Geometry: final body of the model. Coordinates: model frame, mm. A direction names the side the tool comes from. Give positions to 0.01 mm unless a question says otherwise; leave off trailing zeros. Write each loop counter-clockwise with the first axis right and the second up, starting at its lowest first coordinate (ties: lowest second). Pieces come first, ordered by that corner, then holes. Notation, with made-up numbers: M -35,52.25 L -28,52.25 A25 cw -28,91.25 Z; hole C 25,65.25 d11. An arc over 180 degrees is marked long. Answer as a JSON object with one key per item and string values.
from build123d import *

# Parameters (mm, degrees)
F0_W     = 35.56
F0_H     = 35.56
F1_DEPTH = 5.08
F2_W     = 19.812
F2_H     = 4.572
F3_DEPTH = 2.54
F4_W     = 19.812
F4_H     = 4.572
F5_DEPTH = 2.54
F6_W     = 20.32
F6_H     = 5.08
F7_DEPTH = 2.54
F8_W     = 20.32
F8_H     = 5.08
F9_DEPTH = 2.54


with BuildPart() as f1:
    # F0 (on Top) → F1 (new body, symmetric)
    with BuildSketch(Plane.XY):
        Rectangle(F0_W, F0_H)
        Polygon((10.7597222222, 12.4850260417), (10.7597222222, -12.7), (5.4349826389, -12.7), (5.4349826389, -1.8300347222), (-4.5365017361, -1.8300347222), (-4.5365017361, -12.7), (-9.8777777778, -12.7), (-9.8777777778, 12.4850260417), (-4.5365017361, 12.4850260417), (-4.5365017361, 2.6127604167), (5.4349826389, 2.6127604167), (5.4349826389, 12.4850260417), align=None, mode=Mode.SUBTRACT)
    extrude(amount=F1_DEPTH, both=True)

    # F2 (on face) → F3 (join)
    with BuildSketch(Plane(origin=(0, 17.78, 0), x_dir=(-1, 0, 0), z_dir=(0, 1, 0))):
        Rectangle(F2_W, F2_H)
    extrude(amount=F3_DEPTH)

    # F4 (on face) → F5 (join)
    with BuildSketch(Plane(origin=(-17.78, 0, 0), x_dir=(0, -1, 0), z_dir=(-1, 0, 0))):
        Rectangle(F4_W, F4_H)
    extrude(amount=F5_DEPTH)

    # F6 (on face) → F7 (cut)
    with BuildSketch(Plane.XZ.offset(17.78)):
        Rectangle(F6_W, F6_H)
    extrude(amount=-F7_DEPTH, mode=Mode.SUBTRACT)

    # F8 (on face) → F9 (cut)
    with BuildSketch(Plane.YZ.offset(17.78)):
        Rectangle(F8_W, F8_H)
    extrude(amount=-F9_DEPTH, mode=Mode.SUBTRACT)


solid = f1.part
1) Cut plane D-D on y = 8.5. Return loops of the section in (x, z).
Geometry check:
{"outline": "M -20.32,-2.29 L -17.78,-2.29 L -17.78,-5.08 L -9.88,-5.08 L -9.88,5.08 L -17.78,5.08 L -17.78,2.29 L -20.32,2.29 Z; M -4.54,-5.08 L 5.43,-5.08 L 5.43,5.08 L -4.54,5.08 Z; M 10.76,-5.08 L 17.78,-5.08 L 17.78,-2.54 L 15.24,-2.54 L 15.24,2.54 L 17.78,2.54 L 17.78,5.08 L 10.76,5.08 Z"}
2) Cut plane A-A on y = -0.5. Return loops of the section in (x, z), and give its area (3 significant figures).
Geometry check:
{"outline": "M -20.32,-2.29 L -17.78,-2.29 L -17.78,-5.08 L -9.88,-5.08 L -9.88,5.08 L -17.78,5.08 L -17.78,2.29 L -20.32,2.29 Z; M 10.76,-5.08 L 17.78,-5.08 L 17.78,-2.54 L 15.24,-2.54 L 15.24,2.54 L 17.78,2.54 L 17.78,5.08 L 10.76,5.08 Z", "area": "150 mm2"}
3) Pull-direction query (Y, two-part tool) for faces 5 (the flat face through (5.435, 7, 0)), 6 (the flat face through (-9.906, 19, 0)), 7 (the flat face through (0, -15.24, 0)); classes: pulls with the +Y half, pulls with the -Y half, needs draft (parallel to the pull), parting line crosses it, or undercut.
Geometry check:
{"face 5": "undercut", "face 6": "needs draft", "face 7": "pulls with the -Y half"}
4) Set-up query: faces 1 (the flat face through (17, 0, -2.54)), 2 (the flat face through (0, 19, -2.286)), 3 (the flat face through (-19, 0, -2.286)), 4 (the flat face through (0, 2.613, 0)). Return all of +Z, -Z, +X, -X, +Y, -Y with unobstructed straight access to the full face (end or side cutting, diameter ignored); none if empty.
Geometry check:
{"face 1": "+X", "face 2": "-Z, +X, -X, +Y", "face 3": "-Z, -X, +Y, -Y", "face 4": "+Z, -Z"}
5) Cut plane B-B on x = 0.5. Return loops of the section in (y, z).
Geometry check:
{"outline": "M -17.78,-5.08 L -1.83,-5.08 L -1.83,5.08 L -17.78,5.08 L -17.78,2.54 L -15.24,2.54 L -15.24,-2.54 L -17.78,-2.54 Z; M 2.61,-5.08 L 17.78,-5.08 L 17.78,-2.29 L 20.32,-2.29 L 20.32,2.29 L 17.78,2.29 L 17.78,5.08 L 2.61,5.08 Z"}
6) Contact query for flat-ended pins moving along their axis: P1, Ø3, axis at y = -16.5, z = -1, coming from the -X side; P2, Ø1.3, axis at x = -3, y = 19, coming from the +Z side; P3, Ø1.5, axis at y = 1, z = -1, coming from the +X side. Output: stop coordinate, or through.
Geometry check:
{"P1": "stops at x = -17.78", "P2": "stops at z = 2.29", "P3": "stops at x = 15.24"}
7) Line query: line 1 (X direction, y = 9, z = 4.25); line 2 (X direction, y = 4, z = -1.25); line 3 (Y direction, x = 6, z = 0.25). Output: solid intervals per line, ascending. Write a range as from..to.
Geometry check:
{"line 1": "x = -17.78..-9.88, -4.54..5.43, 10.76..17.78", "line 2": "x = -20.32..-9.88, -4.54..5.43, 10.76..15.24", "line 3": "y = -15.24..-12.7, 12.49..20.32"}
